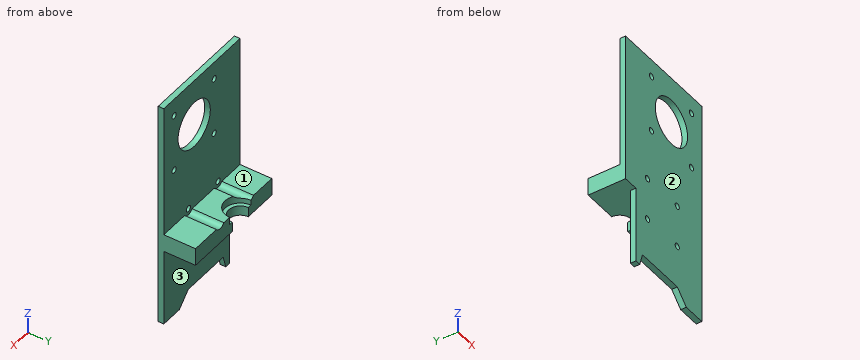
Solid Edge part; units mm, degrees
sketch "Sketch1" plane through (0, 0, 0) normal (0, 1, 0) x (-1, 0, 0)
  circle A0 centre (-11.5, 11.5) radius 1.6
  circle A1 centre (11.5, 11.5) radius 1.6
  circle A2 centre (-11.5, -11.5) radius 1.6
  circle A3 centre (11.5, -11.5) radius 1.6
  circle A4 centre (-7, 56.5) radius 12.5
  circle A5 centre (-22.5, 72) radius 1.6
  circle A6 centre (8.5, 72) radius 1.6
  circle A7 centre (8.5, 41) radius 1.6
  circle A8 centre (-22.5, 41) radius 1.6
  line L0 (20.5, -41.5) -> (17.5, -41.5)
  line L1 (17.5, -41.5) -> (15.4213, -34.5787)
  line L2 (15.4213, -34.5787) -> (-11.5787, -34.5787)
  line L3 (-18.5, -41.5) -> (-11.5787, -34.5787)
  line L4 (-30.5, -41.5) -> (-18.5, -41.5)
  line L5 (-30.5, 81.5) -> (-30.5, -41.5)
  line L6 (28.5, 81.5) -> (-30.5, 81.5)
  line L7 (28.5, 0) -> (28.5, 81.5)
  line L8 (28.5, 0) -> (20.5, 0)
  line L9 (20.5, 0) -> (20.5, -41.5)
  dimension "D1" = 11.5
  dimension "D2" = 11.5
  dimension "D3" = 8.5
  dimension "D4" = 22.5
  dimension "D5" = 28.5
  dimension "D6" = 20.5
extrude "Protrusion1" add sketch "Sketch1" along normal blind 3
sketch "Sketch2" plane through (1, 3, 20) normal (0, 1, 0) x (-1, 0, 0)
  line L0 (15.3723, -10.5) -> (29.5, -10.5)
  line L1 (29.5, -10.5) -> (29.5, -20)
  line L2 (29.5, -20) -> (21.5, -20)
  line L3 (-29.5, -20) -> (21.5, -20)
  line L4 (-29.5, -20) -> (-29.5, -10.5)
  line L5 (-29.5, -10.5) -> (-13.3723, -10.5)
  line L6 (-7.6277, -10.5) -> (9.6277, -10.5)
  arc A0 (15.3723, -10.5) -> (9.6277, -10.5) centre (12.5, -8.5) cw
  arc A1 (-7.6277, -10.5) -> (-13.3723, -10.5) centre (-10.5, -8.5) cw
  dimension "D1" = 29.5
extrude "Protrusion2" add sketch "Sketch2" along normal blind 17
sketch "Sketch3" plane through (1, 20, -16.25) normal (0, 1, 0) x (-1, 0, 0)
  line L0 (13.2911, 25.75) -> (13.2911, 21.55)
  line L1 (13.2911, 21.55) -> (11.2911, 21.55)
  line L2 (11.2911, 21.55) -> (11.2911, 15.75)
  line L3 (11.2911, 15.75) -> (13.3, 15.75)
  line L4 (13.3, 15.75) -> (13.3, 12.25)
  line L5 (13.3, 12.25) -> (17.1, 12.25)
  line L6 (17.1, 12.25) -> (17.1, -19.45)
  line L7 (17.1, -19.45) -> (5.1, -19.45)
  line L8 (13.2911, 25.75) -> (5.1, 25.75)
  dimension "D1" = 17.1
  dimension "D2" = 13.2911
revolve "RevolvedCutout_1" cut sketch "Sketch3" angle 180 about axis through (-4.1, 20, -35.7) along (0, 0, 1)
For this review, take the finished solid that the model builds, in its own axes (mm). Face numbers are marked on the shaded views. A direction names the side the tool comes from. Give positions to 0.01 mm unless a question says otherwise; leave off trailing zeros. Loops run counter-clockwise (first coordinate to the right, second up) from the corner with the lowest first, then second, coordinate; pieces in that order, holes last.
Item 1: Take a section at C-C, the plane y = 1.5. Give the number of separate pieces and of enclosed holes in the cut face, and give its area (3 significant figures).
Item 2: Take a section at B-B, the plane x = 6.5. State the section outline as (y, z) points, and give its area (3 significant figures).
Item 3: Tool access review of the marked faces 1, 2 and 3: name each direction out of +Z, -Z, +X, -X, +Y, -Y from which nothing blocks a thin tool from reaching the whole face with its end or side.
Item 4: For line 1 along Z through (x, y) = (22.5, 2.25); line 2 along Z through (x, y) = (-8.5, 2.25); line 3 along X through (y, z) = (2.25, 72), list the stretches that pass through material, from the lowest coordinate up.
Item 5: Take a section at A-A, the plane x = 22.5. State the section outline as (y, z) points, and give its area (3 significant figures).
Item 6: Insertion check: pin 1 (12 mm diameter, centred on y = 3.5, z = 29.5, fed in from -X); pin 2 (2.5 mm diameter, centred on y = 2, z = -13.5, fed in from -X); pin 3 (2.5 mm diameter, centred on x = -8.5, z = 72, fed in from -Y); pin 4 (1 mm diameter, centred on x = -6, y = 7.5, fed in from -Z). Each pin has a flat end and moves straight along its axis. Give the tip position at first contact, or say it passes through.
Item 7: Take a section at D-D, the plane z = 11.5. State the section outline as (x, y) points.
Calculated:
1. separate pieces: 1
1. enclosed holes: 9
1. area: 6,150 mm2
2. outline: (0, -34.58) - (3, -34.58) - (3, 0) - (20, 0) - (20, 9.5) - (3, 9.5) - (3, 44.01) - (0, 44.01) - close; (0, 68.99) - (3, 68.99) - (3, 81.5) - (0, 81.5) - close
2. area: 435 mm2
3. face 1: +Z, +X, -X, +Y
3. face 2: +Z, -Z, +X, -X, -Y
3. face 3: -Z, +X, -X, +Y
4. line 1: z = -41.5 to 39.4, 42.6 to 70.4, 73.6 to 81.5
4. line 2: z = -34.58 to 39.4, 42.6 to 70.4, 73.6 to 81.5
4. line 3: x = -28.5 to -10.1, -6.9 to 20.9, 24.1 to 30.5
5. outline: (0, -41.5) - (3, -41.5) - (3, 0) - (20, 0) - (20, 9.5) - (3, 9.5) - (3, 39.4) - (0, 39.4) - close; (0, 42.6) - (3, 42.6) - (3, 70.4) - (0, 70.4) - close; (0, 73.6) - (3, 73.6) - (3, 81.5) - (0, 81.5) - close
5. area: 511 mm2
6. pin 1: stops at x = -28.5
6. pin 2: stops at x = -20.5
6. pin 3: passes through
6. pin 4: stops at z = 0
7. outline: (-28.5, 0) - (-13.1, 0) - (-13.1, 3) - (-28.5, 3) - close; (-9.9, 0) - (9.9, 0) - (9.9, 3) - (-9.9, 3) - close; (13.1, 0) - (30.5, 0) - (30.5, 3) - (13.1, 3) - close
